from build123d import *
from OCP.BRepFilletAPI import BRepFilletAPI_MakeChamfer

# Parameters (mm, degrees)
ESQUISSE1_W        = 145
ESQUISSE1_H        = 145
ESQUISSE1_W_2      = 121
ESQUISSE1_H_2      = 121
BOSS_EXTRU_1_DEPTH = 4
CONG_3_R           = 8
CONG_4_R           = 5
CHANFREIN1_SIZE    = 1
CHANFREIN1_SIZE2   = 1.732050808


with BuildPart() as part:
    # Esquisse1 → Boss.-Extru.1 (new body)
    with BuildSketch(Plane.XY):
        with Locations((72.5, 72.5)):
            Rectangle(ESQUISSE1_W, ESQUISSE1_H)
        with Locations((72.5, 72.5)):
            Rectangle(ESQUISSE1_W_2, ESQUISSE1_H_2, mode=Mode.SUBTRACT)
    extrude(amount=BOSS_EXTRU_1_DEPTH)

    # Congé3
    cong_3_edges = [part.edges().sort_by_distance(p)[0] for p in [
        (0, 145, 2),
        (145, 145, 2),
        (145, 0, 2),
        (0, 0, 2),
    ]]
    fillet(cong_3_edges, radius=CONG_3_R)

    # Congé4
    cong_4_edges = [part.edges().sort_by_distance(p)[0] for p in [
        (133, 133, 2),
        (12, 133, 2),
        (12, 12, 2),
        (133, 12, 2),
    ]]
    fillet(cong_4_edges, radius=CONG_4_R)

    # Chanfrein1: one chamfer whose edges measure the first distance from different faces: ONE call of the kernel's chamfer builder (chamfer() names one face for all edges)
    chanfrein1_edges_1 = [part.edges().sort_by_distance(p)[0] for p in [
        (72.5, 145, 0),
        (0, 72.5, 0),
        (145, 72.5, 0),
        (72.5, 0, 0),
        (142.656854249, 2.343145751, 0),
        (2.343145751, 2.343145751, 0),
        (2.343145751, 142.656854249, 0),
        (142.656854249, 142.656854249, 0),
    ]]
    chanfrein1_side_1 = [part.faces().sort_by_distance(p)[0] for p in [
        (72.5, 9.949390335, 0),
    ]]
    chanfrein1_edges_2 = [part.edges().sort_by_distance(p)[0] for p in [
        (72.5, 145, 4),
    ]]
    chanfrein1_side_2 = [part.faces().sort_by_distance(p)[0] for p in [
        (72.5, 145, 2),
    ]]
    chanfrein1_edges_3 = [part.edges().sort_by_distance(p)[0] for p in [
        (145, 72.5, 4),
    ]]
    chanfrein1_side_3 = [part.faces().sort_by_distance(p)[0] for p in [
        (145, 72.5, 2),
    ]]
    chanfrein1_edges_4 = [part.edges().sort_by_distance(p)[0] for p in [
        (0, 72.5, 4),
    ]]
    chanfrein1_side_4 = [part.faces().sort_by_distance(p)[0] for p in [
        (0, 72.5, 2),
    ]]
    chanfrein1_edges_5 = [part.edges().sort_by_distance(p)[0] for p in [
        (72.5, 0, 4),
    ]]
    chanfrein1_side_5 = [part.faces().sort_by_distance(p)[0] for p in [
        (72.5, 0, 2),
    ]]
    chanfrein1_edges_6 = [part.edges().sort_by_distance(p)[0] for p in [
        (142.656854249, 2.343145751, 4),
    ]]
    chanfrein1_side_6 = [part.faces().sort_by_distance(p)[0] for p in [
        (142.656854249, 2.343145751, 2),
    ]]
    chanfrein1_edges_7 = [part.edges().sort_by_distance(p)[0] for p in [
        (2.343145751, 2.343145751, 4),
    ]]
    chanfrein1_side_7 = [part.faces().sort_by_distance(p)[0] for p in [
        (2.343145751, 2.343145751, 2),
    ]]
    chanfrein1_edges_8 = [part.edges().sort_by_distance(p)[0] for p in [
        (2.343145751, 142.656854249, 4),
    ]]
    chanfrein1_side_8 = [part.faces().sort_by_distance(p)[0] for p in [
        (2.343145751, 142.656854249, 2),
    ]]
    chanfrein1_edges_9 = [part.edges().sort_by_distance(p)[0] for p in [
        (142.656854249, 142.656854249, 4),
    ]]
    chanfrein1_side_9 = [part.faces().sort_by_distance(p)[0] for p in [
        (142.656854249, 142.656854249, 2),
    ]]
    chanfrein1_edges_10 = [part.edges().sort_by_distance(p)[0] for p in [
        (72.5, 12, 0),
        (72.5, 12, 4),
    ]]
    chanfrein1_side_10 = [part.faces().sort_by_distance(p)[0] for p in [
        (72.5, 12, 2),
    ]]
    chanfrein1_edges_11 = [part.edges().sort_by_distance(p)[0] for p in [
        (133, 72.5, 0),
        (133, 72.5, 4),
    ]]
    chanfrein1_side_11 = [part.faces().sort_by_distance(p)[0] for p in [
        (133, 72.5, 2),
    ]]
    chanfrein1_edges_12 = [part.edges().sort_by_distance(p)[0] for p in [
        (72.5, 133, 0),
        (72.5, 133, 4),
    ]]
    chanfrein1_side_12 = [part.faces().sort_by_distance(p)[0] for p in [
        (72.5, 133, 2),
    ]]
    chanfrein1_edges_13 = [part.edges().sort_by_distance(p)[0] for p in [
        (12, 72.5, 0),
        (12, 72.5, 4),
    ]]
    chanfrein1_side_13 = [part.faces().sort_by_distance(p)[0] for p in [
        (12, 72.5, 2),
    ]]
    chanfrein1_edges_14 = [part.edges().sort_by_distance(p)[0] for p in [
        (131.535533906, 13.464466094, 0),
        (131.535533906, 13.464466094, 4),
    ]]
    chanfrein1_side_14 = [part.faces().sort_by_distance(p)[0] for p in [
        (131.535533906, 13.464466094, 2),
    ]]
    chanfrein1_edges_15 = [part.edges().sort_by_distance(p)[0] for p in [
        (131.535533906, 131.535533906, 0),
        (131.535533906, 131.535533906, 4),
    ]]
    chanfrein1_side_15 = [part.faces().sort_by_distance(p)[0] for p in [
        (131.535533906, 131.535533906, 2),
    ]]
    chanfrein1_edges_16 = [part.edges().sort_by_distance(p)[0] for p in [
        (13.464466094, 131.535533906, 0),
        (13.464466094, 131.535533906, 4),
    ]]
    chanfrein1_side_16 = [part.faces().sort_by_distance(p)[0] for p in [
        (13.464466094, 131.535533906, 2),
    ]]
    chanfrein1_edges_17 = [part.edges().sort_by_distance(p)[0] for p in [
        (13.464466094, 13.464466094, 0),
        (13.464466094, 13.464466094, 4),
    ]]
    chanfrein1_side_17 = [part.faces().sort_by_distance(p)[0] for p in [
        (13.464466094, 13.464466094, 2),
    ]]
    chanfrein1 = BRepFilletAPI_MakeChamfer(part.part.solid().wrapped)
    for e in chanfrein1_edges_1:
        chanfrein1.Add(CHANFREIN1_SIZE, CHANFREIN1_SIZE2, e.wrapped, chanfrein1_side_1[0].wrapped)  # the first distance lies on this face
    for e in chanfrein1_edges_2:
        chanfrein1.Add(CHANFREIN1_SIZE, CHANFREIN1_SIZE2, e.wrapped, chanfrein1_side_2[0].wrapped)  # the first distance lies on this face
    for e in chanfrein1_edges_3:
        chanfrein1.Add(CHANFREIN1_SIZE, CHANFREIN1_SIZE2, e.wrapped, chanfrein1_side_3[0].wrapped)  # the first distance lies on this face
    for e in chanfrein1_edges_4:
        chanfrein1.Add(CHANFREIN1_SIZE, CHANFREIN1_SIZE2, e.wrapped, chanfrein1_side_4[0].wrapped)  # the first distance lies on this face
    for e in chanfrein1_edges_5:
        chanfrein1.Add(CHANFREIN1_SIZE, CHANFREIN1_SIZE2, e.wrapped, chanfrein1_side_5[0].wrapped)  # the first distance lies on this face
    for e in chanfrein1_edges_6:
        chanfrein1.Add(CHANFREIN1_SIZE, CHANFREIN1_SIZE2, e.wrapped, chanfrein1_side_6[0].wrapped)  # the first distance lies on this face
    for e in chanfrein1_edges_7:
        chanfrein1.Add(CHANFREIN1_SIZE, CHANFREIN1_SIZE2, e.wrapped, chanfrein1_side_7[0].wrapped)  # the first distance lies on this face
    for e in chanfrein1_edges_8:
        chanfrein1.Add(CHANFREIN1_SIZE, CHANFREIN1_SIZE2, e.wrapped, chanfrein1_side_8[0].wrapped)  # the first distance lies on this face
    for e in chanfrein1_edges_9:
        chanfrein1.Add(CHANFREIN1_SIZE, CHANFREIN1_SIZE2, e.wrapped, chanfrein1_side_9[0].wrapped)  # the first distance lies on this face
    for e in chanfrein1_edges_10:
        chanfrein1.Add(CHANFREIN1_SIZE, CHANFREIN1_SIZE2, e.wrapped, chanfrein1_side_10[0].wrapped)  # the first distance lies on this face
    for e in chanfrein1_edges_11:
        chanfrein1.Add(CHANFREIN1_SIZE, CHANFREIN1_SIZE2, e.wrapped, chanfrein1_side_11[0].wrapped)  # the first distance lies on this face
    for e in chanfrein1_edges_12:
        chanfrein1.Add(CHANFREIN1_SIZE, CHANFREIN1_SIZE2, e.wrapped, chanfrein1_side_12[0].wrapped)  # the first distance lies on this face
    for e in chanfrein1_edges_13:
        chanfrein1.Add(CHANFREIN1_SIZE, CHANFREIN1_SIZE2, e.wrapped, chanfrein1_side_13[0].wrapped)  # the first distance lies on this face
    for e in chanfrein1_edges_14:
        chanfrein1.Add(CHANFREIN1_SIZE, CHANFREIN1_SIZE2, e.wrapped, chanfrein1_side_14[0].wrapped)  # the first distance lies on this face
    for e in chanfrein1_edges_15:
        chanfrein1.Add(CHANFREIN1_SIZE, CHANFREIN1_SIZE2, e.wrapped, chanfrein1_side_15[0].wrapped)  # the first distance lies on this face
    for e in chanfrein1_edges_16:
        chanfrein1.Add(CHANFREIN1_SIZE, CHANFREIN1_SIZE2, e.wrapped, chanfrein1_side_16[0].wrapped)  # the first distance lies on this face
    for e in chanfrein1_edges_17:
        chanfrein1.Add(CHANFREIN1_SIZE, CHANFREIN1_SIZE2, e.wrapped, chanfrein1_side_17[0].wrapped)  # the first distance lies on this face
    add(Compound.cast(chanfrein1.Shape()), mode=Mode.REPLACE)


solid = part.part
Read the model definition and answer for the solid it produces. Units are mm, in the model's axes. A direction names the side the tool comes from. Round coordinates to 2 decimals unless told otherwise and drop trailing zeros. Write each loop counter-clockwise with the first axis right and the second up, starting at its lowest first coordinate (ties: lowest second). Pieces come first, ordered by that corner, then holes.
Q1. Straight lines are drawn through the part: line 1 (X direction, y = 121, z = 1.95); line 2 (Y direction, x = 112, z = 0.75). For each, find the intervals that lie inside material, in ascending order.
Values:
line 1: x = 0 to 12, 133 to 145
line 2: y = 0.57 to 11.57, 133.43 to 144.43
Q2. The mould has two halves that part along Y. Classify faces 1 (the face through (142.09, 142.21, 0.49)), 2 (the face through (8, 74, 0)), 3 (the face through (13.159, 131.927, 0.715)): released by +Y, released by -Y, zero draft, split by the parting line, or undercut.
Values:
face 1: released by +Y
face 2: zero draft
face 3: undercut
Q3. Find section A-A on x = 28.5. Determine the outline of the cut face in (y, z).
Values:
outline: (0, 1.73) - (1, 0) - (10.27, 0) - (12, 1) - (12, 3) - (10.27, 4) - (1.73, 4) - (0, 3) - close; (133, 1) - (134.73, 0) - (144, 0) - (145, 1.73) - (145, 3) - (143.27, 4) - (134.73, 4) - (133, 3) - close
Q4. Flat-ended cylindrical pins translate along their axes: P1, Ø2, axis at x = 101, z = 1.5, coming from the +Y side; P2, Ø1, axis at x = 27.5, z = 1, coming from the +Y side. Find the tip coordinate at first contact, or state that the pin passes through.
Values:
P1: stops at y = 145
P2: stops at y = 144.87
Q5. A tool of negligible diameter and unlimited length cuts with its end or side. For faces 4 (the face through (131.927, 131.841, 0.715)), 5 (the face through (2.281, 2.406, 2.375)), 6 (the face through (141.58, 141.68, 3.84)), 7 (the face through (13.073, 13.159, 3.285)), 8 (the face through (131, 13, 2)), from which of +Z, -Z, +X, -X, +Y, -Y can it reach the whole face along a straight path? Write none if from no direction.
Values:
face 4: -Z
face 5: +Z, -Z, -X, -Y
face 6: +Z, +X, +Y
face 7: +Z
face 8: +Z, -Z
